Here's how the part is built. I have some questions about the finished solid (model axes, mm). A direction names the side the tool comes from. Round coordinates to 2 decimals unless told otherwise and drop trailing zeros. Loops run counter-clockwise (first coordinate to the right, second up) from the corner with the lowest first, then second, coordinate; pieces in that order, holes last. Notation, with made-up numbers: M -11,9 L 25,9 A19 ccw 25,41 Z; hole C 4.5,76.5 d7. An arc over 180 degrees is marked long. Answer as CSV lines item,"result".
```python
from build123d import *

# Parameters (mm, degrees)
F0_R     = 5.602905
F1_DEPTH = 25


with BuildPart() as f1:
    # F0 (on Front) → F1 (new body)
    with BuildSketch(Plane.XZ):
        Polygon((-53.839558, 195.515509), (-153.839558, 195.515509), (-153.839558, -34.484491), (446.160442, -34.484491), (446.160442, 195.515509), (306.160442, 195.515509), (306.160442, 45.515509), (296.160442, 45.515509), (296.160442, 195.515509), (246.160442, 195.515509), (246.160442, 45.515509), (236.160442, 45.515509), (236.160442, 195.515509), (186.160442, 195.515509), (186.160442, 45.515509), (176.160442, 45.515509), (176.160442, 195.515509), (-43.839558, 195.515509), (-43.839558, 45.515509), (-53.839558, 45.515509), align=None)
        with Locations((13.436623, 66.090696)):
            Circle(F0_R, mode=Mode.SUBTRACT)
    extrude(amount=F1_DEPTH)


solid = f1.part
```
1. I want a section at B-B, the plane y = -5.5. Please give me the cut outline in (x, z), and give its area (3 significant figures).
Evaluation:
outline,"M -153.84,-34.48 L 446.16,-34.48 L 446.16,195.52 L 306.16,195.52 L 306.16,45.52 L 296.16,45.52 L 296.16,195.52 L 246.16,195.52 L 246.16,45.52 L 236.16,45.52 L 236.16,195.52 L 186.16,195.52 L 186.16,45.52 L 176.16,45.52 L 176.16,195.52 L -43.84,195.52 L -43.84,45.52 L -53.84,45.52 L -53.84,195.52 L -153.84,195.52 Z; hole C 13.44,66.09 d11.21"
area,"132,000 mm²"
2. Which directions (+Z, -Z, +X, -X, +Y, -Y) give clear straight access to the entire face, cutting with the end or side of a thin tool? Please do faces 1 (the flat face through (236.16, -12, 119)), 2 (the flat face through (212, -12, 195.516)).
Evaluation:
face 1,"+Z, +Y, -Y"
face 2,"+Z, +X, -X, +Y, -Y"
3. If I drill on line 1 (X direction, y = -7.25, z = 174); line 2 (Z direction, x = 177.5, y = -16); line 3 (Z direction, x = 18, y = -22.5), over which ranges is the centre line in solid material (lowest first)? Write a range as [from, to].
Evaluation:
line 1,"x = [-153.84, -53.84], [-43.84, 176.16], [186.16, 236.16], [246.16, 296.16], [306.16, 446.16]"
line 2,"z = [-34.48, 45.52]"
line 3,"z = [-34.48, 62.84], [69.34, 195.52]"
4. For P1, Ø8, axis at x = -49, y = -18, coming from the +Z side, with a flat end and sliding along its axis, tell me the tip position at first contact or that it passes through.
Evaluation:
P1,"stops at z = 45.52"
5. I want a section at A-A, the plane z = 151.5. Please give me the cut outline in (x, y).
Evaluation:
outline,"M -153.84,-25 L -53.84,-25 L -53.84,0 L -153.84,0 Z; M -43.84,-25 L 176.16,-25 L 176.16,0 L -43.84,0 Z; M 186.16,-25 L 236.16,-25 L 236.16,0 L 186.16,0 Z; M 246.16,-25 L 296.16,-25 L 296.16,0 L 246.16,0 Z; M 306.16,-25 L 446.16,-25 L 446.16,0 L 306.16,0 Z"
6. We'd pull the mould along X, two halves only. Please class faces 3 (the flat face through (142, 0, 82)), 4 (the flat face through (306.16, -12, 122)), 5 (the flat face through (446.16, -12, 79)): pulls with the +X half, pulls with the -X half, needs draft (parallel to the pull), parting line crosses it, or undercut.
Evaluation:
face 3,"needs draft"
face 4,"undercut"
face 5,"pulls with the +X half"
